Autodesk Inventor part; units mm, degrees
ref_plane "YZ Plane" through (0, 0, 0) normal (1, 0, 0) x (0, 1, 0)
ref_plane "XZ Plane" through (0, 0, 0) normal (0, 1, 0) x (-1, 0, 0)
ref_plane "XY Plane" through (0, 0, 0) normal (0, 0, 1) x (1, 0, 0)
sketch "Sketch1" plane through (0, 0, 0) normal (0, 1, 0) x (-1, 0, 0)
  line L0 (25, -12.5) -> (-25, -12.5)
  line L1 (-25, -12.5) -> (-25, 12.5)
  line L2 (-25, 12.5) -> (25, 12.5)
  line L3 (25, 12.5) -> (25, -12.5)
  line L4 (25, -12.5) -> (-25, 12.5) construction
  line L5 (-25, -12.5) -> (25, 12.5) construction
  arc A0 (-3.2076, 33.6886) -> (-4, 33.1054) centre (0, 28.5) ccw
  arc A1 (-4, 37.6652) -> (4, 37.6652) centre (0, 28.5) ccw
  line L6 (25, -12.5) -> (-25, -12.5)
  line L7 (-25, -12.5) -> (-25, 7.5)
  line L8 (-25, 7.5) -> (25, 7.5)
  line L9 (25, 7.5) -> (25, -12.5)
  line L10 (0, 28.5) -> (0, 0) construction
  line L11 (10, 28.5) -> (10, 12.5)
  line L12 (-10, 28.5) -> (-10, 12.5)
  line L13 (-4, 44.5) -> (-0.5, 44.5)
  line L14 (4, 44.5) -> (4, 37.6652)
  line L15 (4, 32.5) -> (-4, 32.5) construction
  line L16 (-4, 32.5) -> (-4, 33.1054) construction
  line L17 (-4, 44.5) -> (4, 32.5) construction
  line L18 (4, 44.5) -> (-4, 32.5) construction
  line L19 (0, 28.5) -> (0, 38.5) construction
  line L20 (-4, 37.6652) -> (-4, 44.5)
  line L21 (4, 37.6652) -> (4, 33.1054) construction
  line L22 (4, 33.1054) -> (4, 32.5) construction
  line L23 (-4, 33.1054) -> (-4, 37.6652) construction
  arc A2 (0, 38.5) -> (-4, 37.6652) centre (0, 28.5) ccw construction
  arc A3 (4, 37.6652) -> (0, 38.5) centre (0, 28.5) ccw construction
  arc A4 (0, 34.6) -> (-0.5, 34.5795) centre (0, 28.5) ccw construction
  arc A5 (-4, 33.1054) -> (4, 33.1054) centre (0, 28.5) ccw
  arc A6 (3.2076, 33.6886) -> (0.5, 34.5795) centre (0, 28.5) ccw
  arc A7 (4, 33.1054) -> (3.2076, 33.6886) centre (0, 28.5) ccw
  line L24 (0.5, 44.5) -> (0.5, 34.5795)
  line L25 (-0.5, 44.5) -> (-0.5, 34.5795)
  line L26 (0.5, 44.5) -> (4, 44.5)
  line L27 (-0.5, 44.5) -> (0.5, 44.5) construction
  arc A8 (0.5, 34.5795) -> (0, 34.6) centre (0, 28.5) ccw construction
  arc A9 (-0.5, 34.5795) -> (-3.2076, 33.6886) centre (0, 28.5) ccw
  line L28 (25, -12.5) -> (-25, 7.5) construction
  line L29 (-25, -12.5) -> (25, 7.5) construction
  line L30 (25, -2.5) -> (0, -2.5) construction
  line L31 (0, -2.5) -> (-25, -2.5) construction
  circle A10 centre (0, -2.5) radius 2.5
  circle A11 centre (15, -2.5) radius 2.5
  circle A12 centre (-15, -2.5) radius 2.5
  dimension "d1" = 25
  dimension "d3" = 20
  dimension "d5" = 20
  dimension "d6" = 21
  dimension "d7" = 50
  dimension "d8" = 8
  dimension "d9" = 12
  dimension "d10" = 0.5
  dimension "d12" = 0.5
  dimension "d18" = 5
  dimension "d19" = 5
  dimension "d20" = 5
  dimension "d21" = 10
  dimension "d22" = 10
  dimension "d41" = 6.1
extrude "Extrusion1" add sketch "Sketch1" against normal blind 5 contours L0 L1 L8 L3
extrude "Extrusion2" add sketch "Sketch1" against normal blind 25 contours L8 L1 L2 L3 | L2 L12 A1 L11 | A1 L20 L13 L25 A9 A0 A5 A7 A6 L24 L26 L14
sketch "Sketch2" plane through (25, -5, 7.5) normal (0, 0, -1) x (-1, 0, 0)
  line L0 (0, -20) -> (15, -20)
  line L1 (50, 0) -> (0, 0)
  line L2 (0, 0) -> (0, -20)
  line L3 (0, -20) -> (50, -20)
  line L4 (50, -20) -> (50, 0)
  line L5 (0, 5) -> (0, -20) construction
  line L6 (0, -10) -> (50, -10) construction
  circle A0 centre (7.5, -10) radius 2.5
  circle A1 centre (42.5, -10) radius 2.5
  point P0 (25, 5)
  dimension "d26" = 5
  dimension "d27" = 7.5
  dimension "d28" = 5
  dimension "d29" = 7.5
extrude "Extrusion3" cut sketch "Sketch2" against normal blind 5 contours A0 | A1
sketch "Sketch3" plane through (4, 0, 44.5) normal (1, 0, 0) x (0, 0, -1)
  line L0 (0, 0) -> (0, -25) construction
  line L1 (6.8348, 0) -> (6.8348, -25) construction
  line L2 (0, 0) -> (6.8348, 0) construction
  line L3 (6.8348, 0) -> (6.8348, -25) construction
  line L4 (6.8348, -25) -> (0, -25) construction
  line L5 (0, -25) -> (0, 0) construction
  line L6 (6.8348, -25) -> (0, -25) construction
  line L7 (0, 0) -> (6.8348, -25) construction
  line L8 (0, 0) -> (6.8348, 0) construction
  line L9 (0, -25) -> (6.8348, 0) construction
  line L10 (3.4174, 0) -> (3.4174, -12.5) construction
  line L11 (3.4174, -12.5) -> (3.4174, -25) construction
  circle A0 centre (3.4174, -12.5) radius 1.575
  circle A1 centre (3.4174, -5) radius 1.575
  circle A2 centre (3.4174, -20) radius 1.575
  point P0 (44.5, 0)
  dimension "d32" = 3.15
  dimension "d33" = 3.15
  dimension "d34" = 3.15
  dimension "d35" = 5
  dimension "d36" = 5
extrude "Extrusion4" cut sketch "Sketch3" against normal blind 8
fillet "Fillet1" radius 1 40 edges at (-25, -12.5, 12.5) (-25, -15, 7.5) (-25, -5, -2.5) (-25, 0, 0) (-17.5, 0, 12.5) (-8.3666, 0, 33.9772) (-10, 0, 20.5) (-10, -12.5, 12.5) (-4, -12.5, 37.6652) (-4, 0, 41.0826) (-4, -12.5, 44.5) (-4, -25, 41.0826) (-10, -25, 20.5) (-8.3666, -25, 33.9772) (-17.5, -25, 12.5) (0, -25, 7.5) (-2.25, 0, 44.5) (2.25, 0, 44.5) (4, 0, 41.0826) (10, 0, 20.5) (8.3666, 0, 33.9772) (10, -25, 20.5) (8.3666, -25, 33.9772) (-2.25, -25, 44.5) (2.25, -25, 44.5) (4, -12.5, 44.5) (4, -25, 41.0826) (17.5, -25, 12.5) (25, -12.5, 12.5) (17.5, 0, 12.5) (25, 0, 0) (0, 0, -12.5) (25, -2.5, -12.5) (0, -5, -12.5) (25, -5, -2.5) (25, -15, 7.5) (25, -25, 10) (-25, -2.5, -12.5) (-25, -25, 10) (4, -12.5, 37.6652)
equation "\"d10\" = d12"
properties part number "z_rod_holder" material "Plastic, Opaque Black"
CAD build for the part. Positions are in the model's coordinates, mm. A direction names the side the tool comes from. Coordinates: 2 decimals unless noted, no trailing zeros. Write each loop counter-clockwise with the first axis right and the second up, starting at its lowest first coordinate (ties: lowest second). Pieces come first, ordered by that corner, then holes. Notation, with made-up numbers: (68.5, 3.25) -> (81.5, 3.25) arc R20 ccw to (81.5, 8.25) -> close; hole circle Ø6 at (13, 59.5). An arc over 180 degrees is marked (long way). Use CSV: the item, a comma, the result in double quotes. Start each with the question number.
Item 1: Tool access for faces 4 (the flat face through (-10, -12, 21)), 5 (the cylindrical face through (-1.926, -12.325, 34.288)), 6 (the flat face through (4, -12, 39)), 7 (the flat face through (0.5, -12, 39)): list every direction of +Z, -Z, +X, -X, +Y, -Y with a clear straight run to the whole face (end or side of a thin tool).
Item 2: Drop flat-ended pins along their axis: P1, Ø15, axis at x = 1, y = -15.5, coming from the -Z side; P2, Ø8, axis at x = -15, y = -9.5, coming from the +Z side; P3, Ø8, axis at x = -13.5, z = 0.5, coming from the -Y side; P4, Ø3, axis at x = -5.5, z = 22, coming from the +Y side. Give the stop position or say it passes through.
Item 3: Band-saw the part on B-B, the plane z = 4. Write the cut outline in (x, y).
Item 4: Band-saw the part on A-A, the plane x = 14. Write the cut outline in (y, z).
Item 5: Band-saw the part on C-C, the plane y = -15. Give the number of separate pieces and of enclosed holes in the cut face, plus the area to 3 significant figures.
Item 6: Wall check: probe 1 along Z at (x, y) = (0, -2.75); probe 2 along Y at (x, z) = (-17.5, 10.05); probe 3 along Z at (x, y) = (19.5, -9.75). Give the ranges that are in metal, low to high.
Item 7: Two-plate mould, pull along Y, no slides. Class faces 1 (the cylindrical face through (-2.226, -12.431, 42.656)), 2 (the flat face through (0.3, -5, 0.2)), 3 (the flat face through (2, -12, 44.5)): +Y half, -Y half, draft (parallel to the pull), parting line (faces both ways), or undercut.
Response values:
1,face 4,"+Z, -X, +Y, -Y"
1,face 5,"+Y, -Y"
1,face 6,"+Z, +X, +Y, -Y"
1,face 7,"+Z, +Y, -Y"
2,P1,"stops at z = 7.5"
2,P2,"stops at z = 12.5"
2,P3,"stops at y = -5"
2,P4,"stops at y = 0"
3,outline,"(-25, -4) arc R1 ccw to (-24, -5) -> (24, -5) arc R1 ccw to (25, -4) -> (25, -1) arc R1 ccw to (24, 0) -> (-24, 0) arc R1 ccw to (-25, -1) -> close"
4,outline,"(-25, 8.5) arc R1 ccw to (-24, 7.5) -> (-5, 7.5) -> (-5, -0.21) -> (0, -0.21) -> (0, 11.5) arc R1 ccw to (-1, 12.5) -> (-24, 12.5) arc R1 ccw to (-25, 11.5) -> close; (-5, -11.5) arc R1 ccw to (-4, -12.5) -> (-1, -12.5) arc R1 ccw to (0, -11.5) -> (0, -4.79) -> (-5, -4.79) -> close"
5,separate pieces,"3"
5,enclosed holes,"0"
5,area,"600 mm2"
6,probe 1,"z = -12.5 to -5, 0 to 22.4"
6,probe 2,"y = -25 to -17.5, -12.5 to 0"
6,probe 3,"z = 7.5 to 12.5"
7,face 1,"undercut"
7,face 2,"-Y half"
7,face 3,"draft"
